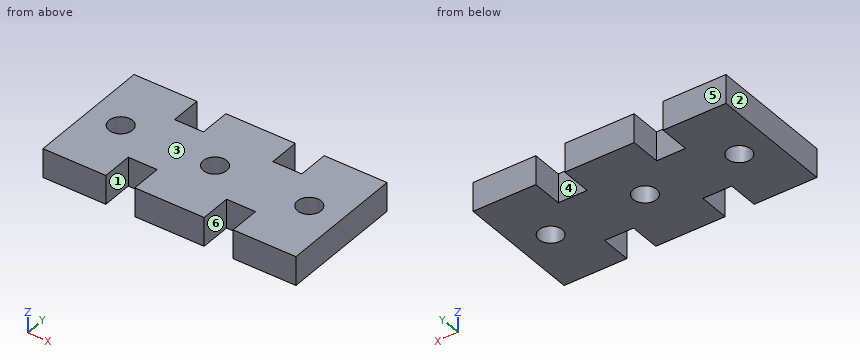
```python
from build123d import *

# Parameters (mm, degrees)
SKETCH1_R           = 2.38125
BOSS_EXTRUDE1_DEPTH = 5.842


with BuildPart() as part:
    # Sketch1 → Boss-Extrude1 (new body)
    with BuildSketch(Plane.XY):
        Polygon((25.5540002, -12.7), (12.8540002, -12.7), (12.8540002, -6.45), (7.0120002, -6.45), (7.0120002, -12.7), (-7.0120002, -12.7), (-7.0120002, -6.45), (-12.8540002, -6.45), (-12.8540002, -12.7), (-25.5540002, -12.7), (-25.5540002, 12.7), (-12.8540002, 12.7), (-12.8540002, 6.45), (-7.0120002, 6.45), (-7.0120002, 12.7), (7.0120002, 12.7), (7.0120002, 6.45), (12.8540002, 6.45), (12.8540002, 12.7), (25.5540002, 12.7), align=None)
        Circle(SKETCH1_R, mode=Mode.SUBTRACT)
        with Locations((-19.05, 0)):
            Circle(SKETCH1_R, mode=Mode.SUBTRACT)
        with Locations(Location((19.05, 0, 0), (0, 0, 180))):
            Circle(SKETCH1_R, mode=Mode.SUBTRACT)
    extrude(amount=BOSS_EXTRUDE1_DEPTH)


solid = part.part
```
Could you check a few things on this model? Use its own coordinates, in mm. Face numbers are marked on the shaded views. A direction names the side the tool comes from. Coordinates: 2 decimals unless noted, no trailing zeros. Write each loop counter-clockwise with the first axis right and the second up, starting at its lowest first coordinate (ties: lowest second). Pieces come first, ordered by that corner, then holes. Notation, with made-up numbers: (54, 31.25) -> (82, 31.25) arc R12 ccw to (82, 48.25) -> close; hole circle Ø2 at (-4.75, 79.5). An arc over 180 degrees is marked (long way). Return JSON: item names as keys, results as strings.
(1) Imagine slicing it at A-A, the plane y = 9.25. Please give me the cut outline in (x, z), then the cut area to 3 significant figures.
Numbers:
{"outline": "(-25.55, 0) -> (-12.85, 0) -> (-12.85, 5.84) -> (-25.55, 5.84) -> close; (-7.01, 0) -> (7.01, 0) -> (7.01, 5.84) -> (-7.01, 5.84) -> close; (12.85, 0) -> (25.55, 0) -> (25.55, 5.84) -> (12.85, 5.84) -> close", "area": "230 mm2"}
(2) Imagine slicing it at B-B, the plane x = 19.05. Please give me the cut outline in (y, z).
Numbers:
{"outline": "(-12.7, 0) -> (-2.38, 0) -> (-2.38, 5.84) -> (-12.7, 5.84) -> close; (2.38, 0) -> (12.7, 0) -> (12.7, 5.84) -> (2.38, 5.84) -> close"}
(3) I'm going to push flat-ended pins straight in: pin 1 (1.5 mm diameter, centred on x = 18.5, y = 0, fed in from +Z); pin 2 (1.5 mm diameter, centred on x = 9, z = 4, fed in from +Y). Where does each tip first touch, or does it pass through?
Numbers:
{"pin 1": "passes through", "pin 2": "stops at y = 6.45"}
(4) Which directions (+Z, -Z, +X, -X, +Y, -Y) give clear straight access to the entire face, cutting with the end or side of a thin tool? Please do the marked faces 4, 5 and 6.
Numbers:
{"face 4": "+Z, -Z, +Y", "face 5": "+Z, -Z, +X, -X, +Y", "face 6": "+Z, -Z, -Y"}
(5) I need wall thicknesses on L1, parallel to X at y = 9.75, z = 3.05; L2, parallel to Y at x = -19.05, z = 3.5; L3, parallel to Y at x = 10, z = 1.9. Which ranges of each line are inside material? Lowest first, please.
Numbers:
{"L1": "x = -25.55 to -12.85, -7.01 to 7.01, 12.85 to 25.55", "L2": "y = -12.7 to -2.38, 2.38 to 12.7", "L3": "y = -6.45 to 6.45"}
(6) We'd pull the mould along X, two halves only. Please class the marked faces 1, 2 and 3: +X half, -X half, draft (parallel to the pull), parting line (faces both ways), or undercut.
Numbers:
{"face 1": "undercut", "face 2": "-X half", "face 3": "draft"}
(7) Imagine slicing it at C-C, the plane y = 0. Please give me the cut outline in (x, z), then the cut area to 3 significant figures.
Numbers:
{"outline": "(-25.55, 0) -> (-21.43, 0) -> (-21.43, 5.84) -> (-25.55, 5.84) -> close; (-16.67, 0) -> (-2.38, 0) -> (-2.38, 5.84) -> (-16.67, 5.84) -> close; (2.38, 0) -> (16.67, 0) -> (16.67, 5.84) -> (2.38, 5.84) -> close; (21.43, 0) -> (25.55, 0) -> (25.55, 5.84) -> (21.43, 5.84) -> close", "area": "215 mm2"}
(8) Imagine slicing it at D-D, the plane z = 3.9. Please give me the cut outline in (x, y), then the cut area to 3 significant figures.
Numbers:
{"outline": "(-25.55, -12.7) -> (-12.85, -12.7) -> (-12.85, -6.45) -> (-7.01, -6.45) -> (-7.01, -12.7) -> (7.01, -12.7) -> (7.01, -6.45) -> (12.85, -6.45) -> (12.85, -12.7) -> (25.55, -12.7) -> (25.55, 12.7) -> (12.85, 12.7) -> (12.85, 6.45) -> (7.01, 6.45) -> (7.01, 12.7) -> (-7.01, 12.7) -> (-7.01, 6.45) -> (-12.85, 6.45) -> (-12.85, 12.7) -> (-25.55, 12.7) -> close; hole circle Ø4.76 at (-19.05, 0); hole circle Ø4.76 at (0, 0); hole circle Ø4.76 at (19.05, 0)", "area": "1,100 mm2"}
